```python
from build123d import *

# Parameters (mm, degrees)
SKETCH1_W           = 381
SKETCH1_H           = 101.6
BOSS_EXTRUDE1_DEPTH = 6.35
SKETCH2_W           = 19.05
SKETCH2_H           = 6.35
SKETCH2_W_2         = 6.35
SKETCH2_H_2         = 12.7
SKETCH2_W_3         = 25.4
CUT_EXTRUDE1_DEPTH  = 6.35
SKETCH3_W           = 50.8
SKETCH3_H           = 63.5
CUT_EXTRUDE2_DEPTH  = 6.35
SKETCH4_W           = 25.4
SKETCH4_H           = 31.75
CUT_EXTRUDE3_DEPTH  = 6.35


with BuildPart() as part:
    # Sketch1 → Boss-Extrude1 (new body)
    with BuildSketch(Plane.XY):
        Rectangle(SKETCH1_W, SKETCH1_H)
    extrude(amount=BOSS_EXTRUDE1_DEPTH)

    # Sketch2 → Cut-Extrude1 (cut)
    with BuildSketch(Plane.XY.offset(6.35)):
        with Locations((-174.625, 47.625)):
            Rectangle(SKETCH2_W, SKETCH2_H)
        with Locations((-187.325, 47.625)):
            Rectangle(SKETCH2_W_2, SKETCH2_H)
        with Locations((-187.325, 41.275)):
            Rectangle(SKETCH2_W_2, SKETCH2_H)
        with Locations((-187.325, 19.05)):
            Rectangle(SKETCH2_W_2, SKETCH2_H_2)
        with Locations((-187.325, -6.35)):
            Rectangle(SKETCH2_W_2, SKETCH2_H_2)
        with Locations((-187.325, -31.75)):
            Rectangle(SKETCH2_W_2, SKETCH2_H_2)
        with Locations((-177.8, -47.625)):
            Rectangle(SKETCH2_W_3, SKETCH2_H)
        with Locations((-127, -47.625)):
            Rectangle(SKETCH2_W_3, SKETCH2_H)
        with Locations((-76.2, -47.625)):
            Rectangle(SKETCH2_W_3, SKETCH2_H)
        with Locations((-25.4, -47.625)):
            Rectangle(SKETCH2_W_3, SKETCH2_H)
        with Locations((25.4, -47.625)):
            Rectangle(SKETCH2_W_3, SKETCH2_H)
        with Locations((-127, 47.625)):
            Rectangle(SKETCH2_W_3, SKETCH2_H)
        with Locations((-76.2, 47.625)):
            Rectangle(SKETCH2_W_3, SKETCH2_H)
        with Locations((-25.4, 47.625)):
            Rectangle(SKETCH2_W_3, SKETCH2_H)
        with Locations((25.4, 47.625)):
            Rectangle(SKETCH2_W_3, SKETCH2_H)
        with Locations((76.2, 47.625)):
            Rectangle(SKETCH2_W_3, SKETCH2_H)
        with Locations((76.2, -47.625)):
            Rectangle(SKETCH2_W_3, SKETCH2_H)
        with Locations((127, -47.625)):
            Rectangle(SKETCH2_W_3, SKETCH2_H)
        with Locations((127, 47.625)):
            Rectangle(SKETCH2_W_3, SKETCH2_H)
        with Locations((174.625, 47.625)):
            Rectangle(SKETCH2_W, SKETCH2_H)
        with Locations((187.325, 47.625)):
            Rectangle(SKETCH2_W_2, SKETCH2_H)
        with Locations((187.325, 41.275)):
            Rectangle(SKETCH2_W_2, SKETCH2_H)
        with Locations((187.325, 19.05)):
            Rectangle(SKETCH2_W_2, SKETCH2_H_2)
        with Locations((187.325, -6.35)):
            Rectangle(SKETCH2_W_2, SKETCH2_H_2)
        with Locations((187.325, -31.75)):
            Rectangle(SKETCH2_W_2, SKETCH2_H_2)
        with Locations((177.8, -47.625)):
            Rectangle(SKETCH2_W_3, SKETCH2_H)
    extrude(amount=-CUT_EXTRUDE1_DEPTH, mode=Mode.SUBTRACT)

    # Sketch3 → Cut-Extrude2 (cut)
    with BuildSketch(Plane.XY.offset(6.35)):
        with Locations((-139.7, -19.05)):
            Rectangle(SKETCH3_W, SKETCH3_H)
        with Locations((139.7, -19.05)):
            Rectangle(SKETCH3_W, SKETCH3_H)
    extrude(amount=-CUT_EXTRUDE2_DEPTH, mode=Mode.SUBTRACT)

    # Sketch4 → Cut-Extrude3 (cut)
    with BuildSketch(Plane.XY.offset(6.35)):
        with Locations((0, 34.925)):
            Rectangle(SKETCH4_W, SKETCH4_H)
    extrude(amount=-CUT_EXTRUDE3_DEPTH, mode=Mode.SUBTRACT)


solid = part.part
```
Verification items for the finished model (mm, model axes). A direction names the side the tool comes from. Give positions to 0.01 mm unless a question says otherwise; leave off trailing zeros. Order: outer loops, then holes, each group sorted by start corner. A loop starts at its lowest first (then second) coordinate and runs counter-clockwise, first axis right, second up. Notation, with made-up numbers: M 62.5,-33.5 L 101.5,-33.5 A24 ccw 101.5,-23.5 Z; hole C -38.5,87 d2. An arc over 180 degrees is marked long. Answer in a Markdown table with one row per item. Add a question column.
Item 1: Scan lines: probe 1 along X at (y, z) = (-42.5, 4); probe 2 along X at (y, z) = (-6, 0.5); probe 3 along X at (y, z) = (23, 5.75). Record each from-to range of solid material in increasing order. Write a range as from..to.
Item 2: Section check A-A, the plane y = -31. Enter the section's corners in (x, z).
Item 3: Section check C-C, the plane x = -159. Enter the section's corners in (y, z).
Item 4: Tool access check on faces 5 (the flat face through (187, -25.4, 3)), 6 (the flat face through (-12.7, -48, 3)), 7 (the flat face through (-102, 50.8, 3)), 8 (the flat face through (-165.1, 48, 3)), 9 (the flat face through (12.7, 32, 3)). Record the directions out of +Z, -Z, +X, -X, +Y, -Y that give a thin tool (end or side, any length) a straight path to the whole face; none if there is none.
Item 5: Gauge pin test, flat ends, axial feed: pin 1 (1.9 mm diameter, centred on y = 48.5, z = 3, fed in from -X); pin 2 (3 mm diameter, centred on x = 133, z = 3.5, fed in from +Y); pin 3 (3 mm diameter, centred on y = 40.5, z = 1.5, fed in from +X). Record the tip position at first contact, or that the pin passes through.
Item 6: Mould release check, pull along Y, two halves, no side actions. Record for faces 1 (the flat face through (190.5, 32, 3)), 2 (the flat face through (187, -12.7, 3)), 3 (the flat face through (-127, 44.45, 3)), 4 (the flat face through (187, -38.1, 3)): released by +Y, released by -Y, zero draft, split by the parting line, or undercut.
Item 7: Section check B-B, the plane x = -83. Enter the section's corners in (y, z), and give its area (3 significant figures).
Filled sheet:
| question | item | result |
|---|---|---|
| 1 | probe 1 | x = -190.5..-165.1, -114.3..114.3, 165.1..190.5 |
| 1 | probe 2 | x = -184.15..-165.1, -114.3..114.3, 165.1..184.15 |
| 1 | probe 3 | x = -184.15..-12.7, 12.7..184.15 |
| 2 | outline | M -184.15,0 L -165.1,0 L -165.1,6.35 L -184.15,6.35 Z; M -114.3,0 L 114.3,0 L 114.3,6.35 L -114.3,6.35 Z; M 165.1,0 L 184.15,0 L 184.15,6.35 L 165.1,6.35 Z |
| 3 | outline | M 12.7,0 L 50.8,0 L 50.8,6.35 L 12.7,6.35 Z |
| 4 | face 5 | +Z, -Z, +X |
| 4 | face 6 | +Z, -Z, -Y |
| 4 | face 7 | +Z, -Z, +X, -X, +Y |
| 4 | face 8 | +Z, -Z, -X, +Y |
| 4 | face 9 | +Z, -Z, +Y |
| 5 | pin 1 | stops at x = -165.1 |
| 5 | pin 2 | stops at y = 44.45 |
| 5 | pin 3 | stops at x = 184.15 |
| 6 | face 1 | zero draft |
| 6 | face 2 | undercut |
| 6 | face 3 | released by +Y |
| 6 | face 4 | undercut |
| 7 | outline | M -44.45,0 L 44.45,0 L 44.45,6.35 L -44.45,6.35 Z |
| 7 | area | 565 mm^2 |
